Autodesk Inventor part; units mm, degrees
ref_plane "YZ Plane" through (0, 0, 0) normal (1, 0, 0) x (0, 1, 0)
ref_plane "XY Plane" through (0, 0, 0) normal (0, 0, 1) x (1, 0, 0)
ref_plane "作業平面2" through (0, 6, 0) normal (0, 1, 0) x (-1, 0, 0)
sketch "スケッチ3" plane through (0, 6, 0) normal (0, 1, 0) x (-1, 0, 0)
  line L0 (4.1, -4.1) -> (-4.1, -4.1)
  line L1 (-4.1, -4.1) -> (-4.1, 4.1)
  line L2 (-4.1, 4.1) -> (4.1, 4.1)
  line L3 (4.1, 4.1) -> (4.1, -4.1)
  line L4 (4.1, -4.1) -> (-4.1, 4.1) construction
  line L5 (-4.1, -4.1) -> (4.1, 4.1) construction
  line L6 (4.875, -4.875) -> (-4.875, -4.875)
  line L7 (-4.875, -4.875) -> (-4.875, 4.875)
  line L8 (-4.875, 4.875) -> (4.875, 4.875)
  line L9 (4.875, 4.875) -> (4.875, -4.875)
  line L10 (4.875, -4.875) -> (-4.875, 4.875) construction
  line L11 (-4.875, -4.875) -> (4.875, 4.875) construction
  point P0 (0, 0)
  point P1 (0, 0)
  dimension "d19" = 8.2
  dimension "d20" = 8.2
  dimension "d21" = 9.75
  dimension "d22" = 9.75
sketch "スケッチ1" plane through (0, 0, 0) normal (0, 1, 0) x (-1, 0, 0)
  line L0 (6.5, -6.5) -> (-6.5, 6.5) construction
  line L1 (-6.5, -6.5) -> (6.5, 6.5) construction
  line L2 (1.046, 3.9037) -> (3.9037, 1.046)
  line L3 (3.9037, 1.046) -> (2.8577, -2.8577)
  line L4 (2.8577, -2.8577) -> (-1.046, -3.9037)
  line L5 (-1.046, -3.9037) -> (-3.9037, -1.046)
  line L6 (-3.9037, -1.046) -> (-2.8577, 2.8577)
  line L7 (-2.8577, 2.8577) -> (1.046, 3.9037)
  line L8 (-6.5, -6.5) -> (6.5, -6.5)
  line L9 (6.5, -6.5) -> (6.5, 6.5)
  line L10 (6.5, 6.5) -> (-6.5, 6.5)
  line L11 (-6.5, 6.5) -> (-6.5, -6.5)
  line L12 (-6.5, -6.5) -> (6.5, 6.5) construction
  line L13 (6.5, -6.5) -> (-6.5, 6.5) construction
  circle A0 centre (0, 0) radius 2.05
  dimension "d33" = 7
  dimension "d34" = 13
  dimension "d35" = 13
  dimension "d36" = 4.1
extrude "押し出し8" add sketch "スケッチ1" along normal blind 6 contours L2 L3 L4 L5 L6 L7 | L11 L10 L9 L8 | A0
extrude "押し出し9" cut sketch "スケッチ3" against normal blind 2
extrude "押し出し10" cut sketch "スケッチ1" along normal blind 3.2 contours L2 L3 L4 L5 L6 L7
extrude "押し出し11" cut sketch "スケッチ1" along normal blind 6 contours A0
properties part number "pin_joint_plastic_ver1"
For this review, take the finished solid that the model builds, in its own axes (mm). A direction names the side the tool comes from. Round coordinates to 2 decimals unless told otherwise and drop trailing zeros. Loops run counter-clockwise (first coordinate to the right, second up) from the corner with the lowest first, then second, coordinate; pieces in that order, holes last. Notation, with made-up numbers: (64.25, 19.25) - (84.25, 19.25) arc R27 ccw to (84.25, 42.25) - close; hole circle Ø6 at (78.5, -39.5). An arc over 180 degrees is marked (long way). One line per question, with ' | ' between items.
Q1. The part is to be moulded in two halves that separate along Z. For faces 1 (the flat face through (0, 3, -6.5)), 2 (the flat face through (6.5, 3, 0)), 3 (the flat face through (-0.933, 1.578, -3.373)), say which applies: released by +Z, released by -Z, zero draft, split by the parting line, or undercut.
Taken from the geometry:
face 1: released by -Z | face 2: zero draft | face 3: undercut
Q2. Tool access review of faces 4 (the flat face through (0, 5, -4.875)), 5 (the flat face through (2, 6, 1)), 6 (the flat face through (2, 3.2, 2)): name each direction out of +Z, -Z, +X, -X, +Y, -Y from which nothing blocks a thin tool from reaching the whole face with its end or side.
Taken from the geometry:
face 4: +Y | face 5: +Z, -Z, +X, -X, +Y | face 6: -Y
Q3. Take a section at D-D (z = 0). Give the boundary of the cut face in (x, y) (3 decimals), and give its area (3 significant figures).
Taken from the geometry:
outline: (-6.5, 0) - (-3.623, 0) - (-3.623, 3.2) - (-2.05, 3.2) - (-2.05, 6) - (-4.1, 6) - (-4.1, 4) - (-4.875, 4) - (-4.875, 6) - (-6.5, 6) - close; (2.05, 3.2) - (3.623, 3.2) - (3.623, 0) - (6.5, 0) - (6.5, 6) - (4.875, 6) - (4.875, 4) - (4.1, 4) - (4.1, 6) - (2.05, 6) - close | area: 40.2 mm²
Q4. Take a section at A-A (y = 5.3). Give the boundary of the cut face in (x, z) (3 decimals), and give its area (3 significant figures).
Taken from the geometry:
outline: (-6.5, -6.5) - (6.5, -6.5) - (6.5, 6.5) - (-6.5, 6.5) - close; (-4.1, -4.1) - (4.1, -4.1) - (4.1, 4.1) - (-4.1, 4.1) - close; hole (-4.875, -4.875) - (4.875, -4.875) - (4.875, 4.875) - (-4.875, 4.875) - close; hole circle Ø4.1 at (0, 0) | area: 128 mm²
Q5. Take a section at C-C (x = -1.5). Give the boundary of the cut face in (y, z) (1 decimal), and give its area (3 significant figures).
Taken from the geometry:
outline: (0, -6.5) - (6, -6.5) - (6, -4.9) - (4, -4.9) - (4, -4.1) - (6, -4.1) - (6, -1.4) - (3.2, -1.4) - (3.2, -3.2) - (0, -3.2) - close; (0, 3.4) - (3.2, 3.4) - (3.2, 1.4) - (6, 1.4) - (6, 4.1) - (4, 4.1) - (4, 4.9) - (6, 4.9) - (6, 6.5) - (0, 6.5) - close | area: 45.7 mm²
Q6. Take a section at B-B (y = 2.35). Give the boundary of the cut face in (x, z), and give its area (3 significant figures).
Taken from the geometry:
outline: (-6.5, -6.5) - (6.5, -6.5) - (6.5, 6.5) - (-6.5, 6.5) - close; hole (-3.9, 1.05) - (-2.86, -2.86) - (1.05, -3.9) - (3.9, -1.05) - (2.86, 2.86) - (-1.05, 3.9) - close | area: 127 mm²
Q7. For line 1 along Z through (x, y) = (0, 4.85) (3 decimals); line 2 along X through (y, z) = (4.55, -2.5) (3 decimals); line 3 along Z through (x, y) = (-4.25, 4.05) (3 decimals), list the stretches that pass through material, from the lowest coordinate up. Write a range as [from, to].
Taken from the geometry:
line 1: z = [-6.5, -4.875], [-4.1, -2.05], [2.05, 4.1], [4.875, 6.5] | line 2: x = [-6.5, -4.875], [-4.1, 4.1], [4.875, 6.5] | line 3: z = [-6.5, -4.875], [4.875, 6.5]
